Geometry: final body of the model. Coordinates: model frame, mm. Round coordinates to 2 decimals unless told otherwise and drop trailing zeros. Loops run counter-clockwise (first coordinate to the right, second up) from the corner with the lowest first, then second, coordinate; pieces in that order, holes last. Notation, with made-up numbers: (37, -5) - (82, -5) arc R20 ccw to (82, 21) - close; hole circle Ø2 at (-18, 73). An arc over 180 degrees is marked (long way). Answer as CSV lines item,"result".
from build123d import *

# Parameters (mm, degrees)
BOSS_EXTRUDE1_DEPTH     = 17.78
SKETCH2_R               = 3.914165929
CUT_EXTRUDE1_DEPTH      = 194.058628532
CUT_EXTRUDE1_DEPTH_BACK = 194.058628532
SKETCH3_R               = 2.54
CUT_EXTRUDE2_DEPTH      = 7.62


with BuildPart() as part:
    # Sketch1 → Boss-Extrude1 (new body)
    with BuildSketch(Plane(origin=(0, 0, 0), x_dir=(0, 0, -1), z_dir=(1, 0, 0))):
        with BuildLine():
            Line((65, 1.27), (-65, 1.27))
            ThreePointArc((-65, 1.27), (-160.342068402, -48.593885399), (-192.5, -151.27))
            Line((-192.5, -151.27), (-189.970093401, -151.043786383))
            ThreePointArc((-189.970093401, -151.043786383), (-158.429364067, -50.266130166), (-64.886150372, -1.27))
            Line((-64.886150372, -1.27), (64.886150372, -1.27))
            ThreePointArc((64.886150372, -1.27), (158.429364067, -50.266130166), (189.970093401, -151.043786383))
            Line((189.970093401, -151.043786383), (192.5, -151.27))
            ThreePointArc((192.5, -151.27), (160.342068402, -48.593885399), (65, 1.27))
        make_face()
    extrude(amount=BOSS_EXTRUDE1_DEPTH)

    # Sketch2 → Cut-Extrude1 (cut, two sides)
    with BuildSketch(Plane.XY) as cut_extrude1_sk:
        with Locations((8.89, -137.16)):
            Circle(SKETCH2_R)
    extrude(amount=CUT_EXTRUDE1_DEPTH, mode=Mode.SUBTRACT)
    extrude(cut_extrude1_sk.sketch, amount=-CUT_EXTRUDE1_DEPTH_BACK, mode=Mode.SUBTRACT)

    # Sketch3 → Cut-Extrude2 (cut)
    with BuildSketch(Plane(origin=(0, 1.27, 0), x_dir=(1, 0, 0), z_dir=(0, 1, 0))):
        with Locations((8.89, 38.1)):
            Circle(SKETCH3_R)
        with Locations((8.89, -38.1)):
            Circle(SKETCH3_R)
    extrude(amount=-CUT_EXTRUDE2_DEPTH, mode=Mode.SUBTRACT)


solid = part.part
(1) Section D-D (y = -114). Output: boundary loops of the cut face in (x, z), and give its area (3 significant figures).
Findings below:
outline,"(0, -190.86) - (17.78, -190.86) - (17.78, -188.28) - (0, -188.28) - close; (0, 188.28) - (17.78, 188.28) - (17.78, 190.86) - (0, 190.86) - close"
area,"91.8 mm2"
(2) Section A-A (y = -17.5). Output: boundary loops of the cut face in (x, z), and give its area (3 significant figures).
Findings below:
outline,"(0, -123.62) - (17.78, -123.62) - (17.78, -118.46) - (0, -118.46) - close; (0, 118.46) - (17.78, 118.46) - (17.78, 123.62) - (0, 123.62) - close"
area,"184 mm2"
(3) Section C-C (z = 15.5). Output: boundary loops of the cut face in (x, y), and give its area (3 significant figures).
Findings below:
outline,"(0, -1.27) - (17.78, -1.27) - (17.78, 1.27) - (0, 1.27) - close"
area,"45.2 mm2"
(4) Section B-B (y = -137.16). Output: boundary loops of the cut face in (x, z), and give its area (3 significant figures).
Findings below:
outline,"(0, -193.05) - (4.98, -193.05) - (4.98, -190.51) - (0, -190.51) - close; (0, 190.51) - (4.98, 190.51) - (4.98, 193.05) - (0, 193.05) - close; (12.8, -193.05) - (17.78, -193.05) - (17.78, -190.51) - (12.8, -190.51) - close; (12.8, 190.51) - (17.78, 190.51) - (17.78, 193.05) - (12.8, 193.05) - close"
area,"50.6 mm2"
(5) Pin query (flat end, axial travel): P1, Ø10, axis at x = 8.89, y = -137.16, coming from the +Z side; P2, Ø2, axis at x = 11.5, y = -71.5, coming from the +Z side; P3, Ø10, axis at x = 6.5, z = 127, coming from the +Y side; P4, Ø3, axis at x = 11, z = 11.5, coming from the -Y side. Return the tip coordinate at first contact, or that it passes through.
Findings below:
P1,"z = 193.06"
P2,"z = 176.47"
P3,"y = -16.56"
P4,"y = -1.27"
(6) Material intervals for line 1 along Z through (x, y) = (4, -126.5); line 2 along X through (y, z) = (-137.16, 191.35); line 3 along X through (y, z) = (0, -38), sorted ascending.
Findings below:
line 1,"-192.52 to -189.97, 189.97 to 192.52"
line 2,"0 to 4.98, 12.8 to 17.78"
line 3,"0 to 6.35, 11.43 to 17.78"
(7) Draft query along Z for faces 1 (the face through (8.77, -49.79, -161.33)), 2 (the face through (17.78, -1, 1)), 3 (the face through (9, -1.27, 1)). Return one class per face: pulls with the +Z half, pulls with the -Z half, needs draft (parallel to the pull), parting line crosses it, or undercut.
Findings below:
face 1,"pulls with the -Z half"
face 2,"needs draft"
face 3,"undercut"
